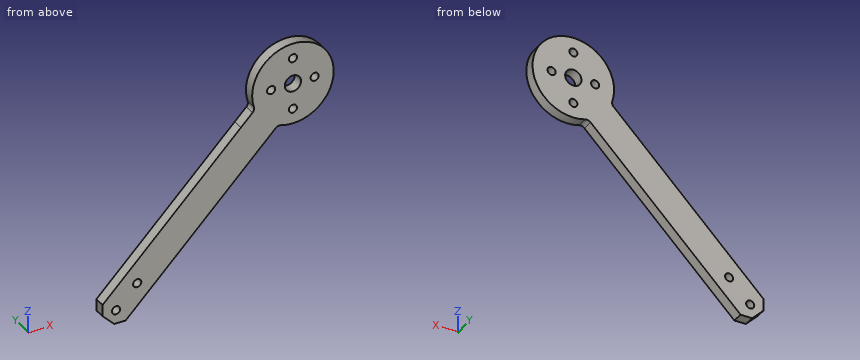
Autodesk Inventor part; units mm, degrees
ref_plane "Motor Simulering" through (0, 14, 0) normal (0, 1, 0) x (1, 0, 0)
ref_plane "YZ Plane" through (0, 0, 0) normal (1, 0, 0) x (0, 1, 0)
ref_plane "XZ Plane" through (0, 0, 0) normal (0, 1, 0) x (-1, 0, 0)
sketch "Sketch1" plane through (0, 0, 0) normal (0, 1, 0) x (-1, 0, 0)
  arc A0 (-76.1755, 50.0335) -> (-86.1582, 40.0508) centre (-90.5256, 54.4009) ccw
  circle A1 centre (-25.4718, -10.6529) radius 1.5
  line L0 (-24.7647, -15.6026) -> (-20.5221, -11.36)
  line L1 (-24.7647, -15.6026) -> (-29.0074, -15.6026)
  line L2 (-20.5221, -11.36) -> (-20.5221, -7.1174)
  circle A2 centre (-33.25, -2.8747) radius 1.5
  circle A3 centre (-90.5256, 44.9009) radius 1.5
  circle A4 centre (-98.5256, 54.4009) radius 1.5
  circle A5 centre (-90.5256, 63.9009) radius 1.5
  circle A6 centre (-82.5256, 54.4009) radius 1.5
  circle A7 centre (-90.5256, 54.4009) radius 3
  arc A8 (-76.1755, 50.0335) -> (-75.6764, 48.037) centre (-74.2622, 49.4512) ccw
  arc A9 (-84.1617, 39.5517) -> (-86.1582, 40.0508) centre (-85.5759, 38.1375) ccw
  line L3 (-75.6764, 48.037) -> (-71.4338, 43.7943)
  line L4 (-84.1617, 39.5517) -> (-79.919, 35.309)
  line L5 (-20.5221, -7.1174) -> (-71.4338, 43.7943)
  line L6 (-29.0074, -15.6026) -> (-79.919, 35.309)
  point P0 (0, 0)
  point P1 (-18.4008, -9.2387)
  point P2 (-76.5619, 48.9225)
  point P3 (-85.0472, 40.4372)
  point P4 (-26.886, -17.724)
  point P5 (-76.5619, 48.9225)
  dimension "d2" = 3
  dimension "d3" = 3
  dimension "d4" = 3
  dimension "d6" = 6
  dimension "d10" = 2
extrude "Extrusion3" add sketch "Sketch1" along normal blind 4
ref_plane "Motor Simulering" through (0, 14, 0) normal (0, 1, 0) x (1, 0, 0)
sketch "Propeller" plane through (0, 14, 0) normal (0, 1, 0) x (1, 0, 0)
  circle A0 centre (90.5256, -54.4009) radius 63.5
  point P0 (0, 0)
  dimension "d26" = 127
properties part number "Arm2"
Verification items for the finished model (mm, model axes). Round coordinates to 2 decimals unless told otherwise and drop trailing zeros. Write each loop counter-clockwise with the first axis right and the second up, starting at its lowest first coordinate (ties: lowest second). Pieces come first, ordered by that corner, then holes.
(1) Section check B-B (y = 2.1). Enter the section's corners in (x, z), plus the area to 3 significant figures.
Returned:
outline: (20.52, -11.36) - (24.76, -15.6) - (29.01, -15.6) - (84.16, 39.55) arc R2 cw to (86.16, 40.05) arc R15 ccw (long way) to (76.18, 50.03) arc R2 cw to (75.68, 48.04) - (71.43, 43.79) - (20.52, -7.12) - close; hole circle Ø3 at (25.47, -10.65); hole circle Ø3 at (33.25, -2.87); hole circle Ø3 at (82.53, 54.4); hole circle Ø6 at (90.53, 54.4); hole circle Ø3 at (90.53, 44.9); hole circle Ø3 at (90.53, 63.9); hole circle Ø3 at (98.53, 54.4)
area: 1,600 mm2
(2) Depth check by flat-ended pin: pin 1 Ø5 at (x, z) = (90.53, 44.9) entering from -Y; pin 2 Ø2 at (y, z) = (1, 20) entering from +X; pin 3 Ø2 at (y, z) = (3, 19.5) entering from -X; pin 4 Ø3.5 at (x, z) = (90.53, 54.4) entering from -Y. Enter the tip coordinate at first touch or a pass-through.
Returned:
pin 1: stops at y = 0
pin 2: stops at x = 65.61
pin 3: stops at x = 46.14
pin 4: passes through
(3) Section check D-D (x = 63). Enter the section's corners in (y, z), plus the area to 3 significant figures.
Returned:
outline: (0, 18.39) - (4, 18.39) - (4, 35.36) - (0, 35.36) - close
area: 67.9 mm2
(4) Material ranges on line 1 (X direction, y = 1.65, z = 53.5); line 2 (X direction, y = 1.2, z = 55); line 3 (Z direction, x = 82.5, y = 3.6), recorded low to high.
Returned:
line 1: x = 75.55 to 81.33, 83.72 to 87.66, 93.39 to 97.33, 99.72 to 105.5
line 2: x = 75.54 to 81.15, 83.9 to 87.59, 93.47 to 97.15, 99.9 to 105.51
line 3: z = 37.89 to 52.9, 55.9 to 67.07
(5) Section check A-A (x = 33.25). Enter the section's corners in (y, z).
Returned:
outline: (0, -11.36) - (4, -11.36) - (4, -4.37) - (0, -4.37) - close; (0, -1.37) - (4, -1.37) - (4, 5.61) - (0, 5.61) - close
(6) Section check C-C (z = 29). Enter the section's corners in (x, y), plus the area to 3 significant figures.
Returned:
outline: (56.64, 0) - (73.61, 0) - (73.61, 4) - (56.64, 4) - close
area: 67.9 mm2
